```python
from build123d import *

# Parameters (mm, degrees)
F0_W     = 990.6
F0_H     = 762
F0_W_2   = 152.4
F0_H_2   = 175.9045571089
F0_H_3   = 181.9028109312
F1_DEPTH = 25.4
F2_R     = 5.08
F3_R     = 5.08
F4_SIZE  = 5.08


with BuildPart() as f1:
    # F0 (on Front) → F1 (new body)
    with BuildSketch(Plane.XZ):
        with Locations((0.8916221559, -189.7441043131)):
            Rectangle(F0_W, F0_H)
        with Locations((-267.8943658352, -87.9522785544)):
            Rectangle(F0_W_2, F0_H_2, mode=Mode.SUBTRACT)
        with Locations((181.9738661766, -90.9514054656)):
            Rectangle(F0_W_2, F0_H_3, mode=Mode.SUBTRACT)
    extrude(amount=F1_DEPTH)

    # F2
    f2_edges = [f1.edges().sort_by_distance(p)[0] for p in [
        (0.891622, -25.4, 191.255896),
    ]]
    fillet(f2_edges, radius=F2_R)

    # F3
    f3_edges = [f1.edges().sort_by_distance(p)[0] for p in [
        (0.891622, -25.4, 186.175896),
        (496.191622, -25.4, -192.284104),
    ]]
    fillet(f3_edges, radius=F3_R)

    # F4
    f4_edges = [f1.edges().sort_by_distance(p)[0] for p in [
        (496.191622, 0, -192.284104),
    ]]
    chamfer(f4_edges, length=F4_SIZE)


solid = f1.part
```
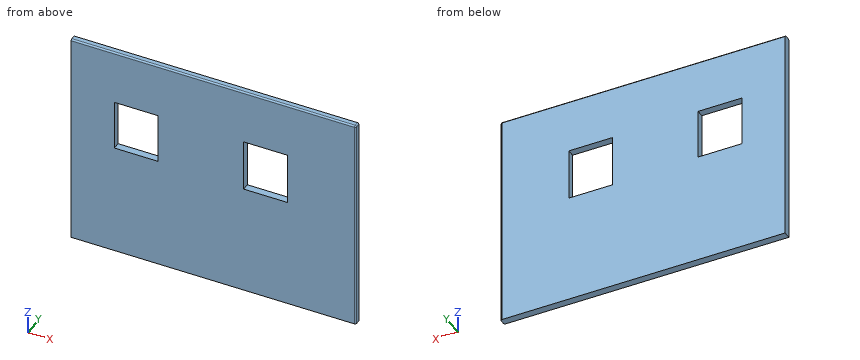
The model under review builds one solid part; all positions refer to its coordinate system, in mm. Coordinates: 2 decimals unless noted, no trailing zeros. Order: outer loops, then holes, each group sorted by start corner. A loop starts at its lowest first (then second) coordinate and runs counter-clockwise, first axis right, second up. Notation, with made-up numbers: (67.5, -20) -> (76.5, -20) arc R29 cw to (76.5, 17) -> close; hole circle Ø8 at (-6.75, 68). An arc over 180 degrees is marked (long way). Answer in a Markdown table with one row per item. Add a question column.
Item 1: We need section A-A on y = -16.5. Write out the cut boundary in (x, z).
Item 2: We need section C-C on z = -62. Write out the cut boundary in (x, y).
Item 3: To check wall thickness, follow probe 1 along X at (y, z) = (-7.5, -50); probe 2 along Z at (x, y) = (-281.5, -16.5); probe 3 along Z at (x, y) = (208.5, -18.5). State the ranges of each line that lie inside material, in increasing order.
Item 4: We need section B-B on x = -244.5. Write out the cut boundary in (y, z).
Item 5: We need section D-D on x = 167.5. Write out the cut boundary in (y, z), plus the area to 3 significant figures.
Final values:
| question | item | result |
|---|---|---|
| 1 | outline | (-494.41, -570.74) -> (496.19, -570.74) -> (496.19, 186.18) arc R5.08 ccw to (491.11, 191.26) -> (-494.41, 191.26) -> close; hole (-344.09, -175.9) -> (-191.69, -175.9) -> (-191.69, 0) -> (-344.09, 0) -> close; hole (105.77, -181.9) -> (258.17, -181.9) -> (258.17, 0) -> (105.77, 0) -> close |
| 2 | outline | (-494.41, -25.4) -> (-344.09, -25.4) -> (-344.09, 0) -> (-494.41, 0) -> close; (-191.69, -25.4) -> (105.77, -25.4) -> (105.77, 0) -> (-191.69, 0) -> close; (258.17, -25.4) -> (491.11, -25.4) arc R5.08 ccw to (496.19, -20.32) -> (496.19, -5.08) -> (491.11, 0) -> (258.17, 0) -> close |
| 3 | probe 1 | x = -494.41 to -344.09, -191.69 to 105.77, 258.17 to 496.19 |
| 3 | probe 2 | z = -570.74 to -175.9, 0 to 191.26 |
| 3 | probe 3 | z = -570.74 to -181.9, 0 to 191.26 |
| 4 | outline | (-25.4, -570.74) -> (0, -570.74) -> (0, -175.9) -> (-25.4, -175.9) -> close; (-25.4, 0) -> (0, 0) -> (0, 186.18) -> (-5.08, 191.26) -> (-20.32, 191.26) arc R5.08 ccw to (-25.4, 186.18) -> close |
| 5 | outline | (-25.4, -570.74) -> (0, -570.74) -> (0, -181.9) -> (-25.4, -181.9) -> close; (-25.4, 0) -> (0, 0) -> (0, 186.18) -> (-5.08, 191.26) -> (-20.32, 191.26) arc R5.08 ccw to (-25.4, 186.18) -> close |
| 5 | area | 14,700 mm2 |
